from build123d import *

# Parameters (mm, degrees)
F0_R     = 21.5
F1_DEPTH = 6
F2_R     = 16.5
F3_DEPTH = 10
F4_R     = 11.125
F5_DEPTH = 8
F6_R     = 9
F7_DEPTH = 8.001
F8_SIZE  = 3


with BuildPart() as f1:
    # F0 (on Front) → F1 (new body)
    with BuildSketch(Plane.XZ):
        Circle(F0_R)
    extrude(amount=-F1_DEPTH)

    # F2 (on face) → F3 (join)
    with BuildSketch(Plane.XZ):
        Circle(F2_R)
    extrude(amount=F3_DEPTH)

    # F4 (on face) → F5 (cut, through all)
    with BuildSketch(Plane(origin=(0, 6, 0), x_dir=(-1, 0, 0), z_dir=(0, 1, 0))):
        Circle(F4_R)
    extrude(amount=-F5_DEPTH, mode=Mode.SUBTRACT)

    # F6 (on face) → F7 (cut, through all)
    with BuildSketch(Plane(origin=(0, -2, 0), x_dir=(-1, 0, 0), z_dir=(0, 1, 0))):
        Circle(F6_R)
    extrude(amount=-F7_DEPTH, mode=Mode.SUBTRACT)

    # F8
    f8_edges = [f1.edges().sort_by_distance(p)[0] for p in [
        (9, -10, 0),
    ]]
    chamfer(f8_edges, length=F8_SIZE)


solid = f1.part
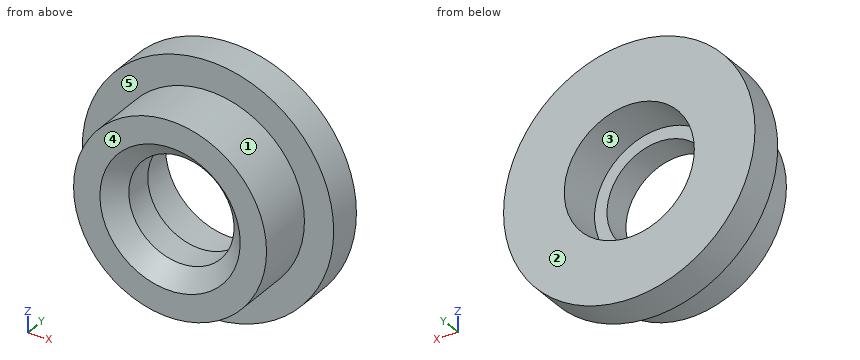
Read the model definition and answer for the solid it produces. Units are mm, in the model's axes. Face numbers are marked on the shaded views. A direction names the side the tool comes from. Round coordinates to 2 decimals unless told otherwise and drop trailing zeros. Loops run counter-clockwise (first coordinate to the right, second up) from the corner with the lowest first, then second, coordinate; pieces in that order, holes last.
Q1. Each of these flat-tipped pins is pushed along its axis until it touches: pin 1 (3 mm diameter, centred on x = 9, y = -1, fed in from +Z); pin 2 (1 mm diameter, centred on y = -5.5, z = -13, fed in from -X); pin 3 (1 mm diameter, centred on x = -5.5, y = 0.5, fed in from -Z); pin 4 (13.5 mm diameter, centred on x = 0, z = 0, fed in from +Y). Where does it stop, or does it pass through?
Q2. Section D-D on z = -14 is taken. Write down the section's boundary in (x, y), and give its area (3 significant figures).
Q3. Section B-B on x = 0 is taken. Write down the section's boundary in (y, z) (3 decimals).
Q4. Determine the mould class of the marked faces 1, 2 and 3 for opening direction Z: released by +Z, released by -Z, zero draft, split by the parting line, or undercut.
Q5. Section A-A on z = 0 is taken. Write down the section's boundary in (x, y) (3 decimals).
Q6. Consider probe 1 along Z at (x, y) = (0, 4.25) (3 decimals); probe 2 along Z at (x, y) = (0, -2.5); probe 3 along X at (y, z) = (-5, -1). Determine where each line is inside the solid, lowest interval first.
Q7. Section C-C on y = -9 is taken. Write down the section's boundary in (x, z).
Q8. Which of the six approach directions +Z, -Z, +X, -X, +Y, -Y give full straight-line access (tool end or side, diameter ignored) to the marked faces 4 and 5?
Output:
1. pin 1: stops at z = 20
1. pin 2: stops at x = -10.77
1. pin 3: stops at z = -20.91
1. pin 4: passes through
2. outline: (-16.32, 0) - (-8.73, 0) - (-8.73, -10) - (8.73, -10) - (8.73, 0) - (16.32, 0) - (16.32, 6) - (-16.32, 6) - close
2. area: 370 mm2
3. outline: (-10, -16.5) - (0, -16.5) - (0, -21.5) - (6, -21.5) - (6, -11.125) - (-2, -11.125) - (-2, -9) - (-7, -9) - (-10, -12) - close; (-10, 12) - (-7, 9) - (-2, 9) - (-2, 11.125) - (6, 11.125) - (6, 21.5) - (0, 21.5) - (0, 16.5) - (-10, 16.5) - close
4. face 1: split by the parting line
4. face 2: zero draft
4. face 3: undercut
5. outline: (-21.5, 0) - (-16.5, 0) - (-16.5, -10) - (-12, -10) - (-9, -7) - (-9, -2) - (-11.125, -2) - (-11.125, 6) - (-21.5, 6) - close; (9, -7) - (12, -10) - (16.5, -10) - (16.5, 0) - (21.5, 0) - (21.5, 6) - (11.125, 6) - (11.125, -2) - (9, -2) - close
6. probe 1: z = -21.5 to -11.125, 11.125 to 21.5
6. probe 2: z = -16.5 to -9, 9 to 16.5
6. probe 3: x = -16.47 to -8.94, 8.94 to 16.47
7. outline: circle Ø33 at (0, 0); hole circle Ø22 at (0, 0)
8. face 4: +Z, -Z, +X, -X, -Y
8. face 5: -Y
